Geometry: final body of the model. Coordinates: model frame, mm. Face numbers are marked on the shaded views. Coordinates: 2 decimals unless noted, no trailing zeros. Answer in a Markdown table with one row per item.
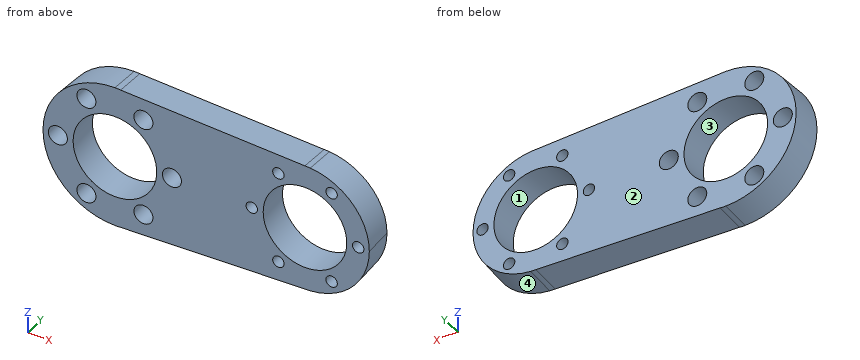
from build123d import *

# Parameters (mm, degrees)
F1_DEPTH = 8
F1_TAPER = -3
F3_D     = 22
F4_D     = 22
F6_D     = 5
F7_D     = 3


# Not quite as in the source:
# - a feature of the source that left no trace in its solid (it failed there, or was rolled back) is left out


with BuildPart() as f1:
    # F0 (on Front) → F1 (new body)
    with BuildSketch(Plane.XZ):
        with BuildLine():
            Line((1.4786393064, 18.4408141307), (0, 18.5))
            ThreePointArc((0, 18.5), (-18.5, 0), (0, -18.5))
            Line((0, -18.5), (1.4786393064, -18.4408141307))
            ThreePointArc((1.4786393064, -18.4408141307), (13.5942051472, -12.5478120171), (18.5, 0))
            ThreePointArc((18.5, 0), (13.5942051472, 12.5478120171), (1.4786393064, 18.4408141307))
        make_face()
        with BuildLine():
            ThreePointArc((1.4786393064, 18.4408141307), (0.7399116781, 18.4851976108), (0, 18.5))
            Line((0, 18.5), (1.4786393064, 18.4408141307))
        make_face()
        with BuildLine():
            Line((1.4786393064, -18.4408141307), (0, -18.5))
            ThreePointArc((0, -18.5), (0.7399116781, -18.4851976108), (1.4786393064, -18.4408141307))
        make_face()
        with BuildLine():
            Line((49.9667920397, 16.4999665827), (1.4786393064, 18.4408141307))
            ThreePointArc((1.4786393064, 18.4408141307), (13.5942051472, 12.5478120171), (18.5, 0))
            Line((18.5, 0), (33.5, 0))
            ThreePointArc((33.5, 0), (38.3210032249, 11.6555151893), (49.9667920397, 16.4999665827))
        make_face()
        with BuildLine():
            ThreePointArc((18.5, 0), (13.5942051472, -12.5478120171), (1.4786393064, -18.4408141307))
            Line((1.4786393064, -18.4408141307), (49.9667920397, -16.4999665827))
            ThreePointArc((49.9667920397, -16.4999665827), (38.3210032249, -11.6555151893), (33.5, 0))
            Line((33.5, 0), (18.5, 0))
        make_face()
        with BuildLine():
            Line((51.3518854576, 16.4445250983), (49.9667920397, 16.4999665827))
            ThreePointArc((49.9667920397, 16.4999665827), (38.3210032249, 11.6555151893), (33.5, 0))
            ThreePointArc((33.5, 0), (38.3210032249, -11.6555151893), (49.9667920397, -16.4999665827))
            Line((49.9667920397, -16.4999665827), (51.3518854576, -16.4445250983))
            ThreePointArc((51.3518854576, -16.4445250983), (62.1358170316, -11.1790851582), (66.5, 0))
            ThreePointArc((66.5, 0), (62.1358170316, 11.1790851582), (51.3518854576, 16.4445250983))
        make_face()
        with BuildLine():
            ThreePointArc((51.3518854576, 16.4445250983), (50.6599212264, 16.4867978691), (49.9667920397, 16.4999665827))
            Line((49.9667920397, 16.4999665827), (51.3518854576, 16.4445250983))
        make_face()
        with BuildLine():
            Line((51.3518854576, -16.4445250983), (49.9667920397, -16.4999665827))
            ThreePointArc((49.9667920397, -16.4999665827), (50.6599212264, -16.4867978691), (51.3518854576, -16.4445250983))
        make_face()
    extrude(amount=F1_DEPTH, taper=F1_TAPER)

    # F3 (through all)
    with Locations(Plane(origin=(0, 0, 0), x_dir=(1, 0, 0), z_dir=(0, 1, 0))):
        with Locations((50, 0)):
            Hole(F3_D / 2)

    # F4 (through all)
    with Locations(Plane(origin=(0, 0, 0), x_dir=(1, 0, 0), z_dir=(0, 1, 0))):
        with Locations((0, 0)):
            Hole(F4_D / 2)

    # F6 (through all)
    with Locations(Plane.XZ.offset(8)):
        with Locations((15, 0), (7.5, 12.9903810568), (-7.5, 12.9903810568), (-15, 0), (-7.5, -12.9903810568), (7.5, -12.9903810568)):
            Hole(F6_D / 2)

    # F7 (through all)
    with Locations(Plane.XZ.offset(8)):
        with Locations((36, 0), (43, 12.124355653), (57, 12.124355653), (64, 0), (57, -12.124355653), (43, -12.124355653)):
            Hole(F7_D / 2)


solid = f1.part
(1) Ray query, probe 1 along Z at (x, y) = (-15, -1.75); probe 2 along Z at (x, y) = (-7.5, -3.75); probe 3 along X at (y, z) = (-5.5, 3). Return the intervals inside material, ascending.
Verdict:
| item | result |
|---|---|
| probe 1 | z = -10.98 to -2.5, 2.5 to 10.98 |
| probe 2 | z = -17.13 to -15.49, -10.49 to -8.05, 8.05 to 10.49, 15.49 to 17.13 |
| probe 3 | x = -18.55 to -10.58, 10.58 to 39.42, 60.58 to 66.52 |
(2) Cut plane A-A on x = 57. State how many separate pieces and enclosed holes the cut face has, then the cut area to 3 significant figures.
Verdict:
| item | result |
|---|---|
| separate pieces | 4 |
| enclosed holes | 0 |
| area | 59.0 mm² |
(3) Pull-direction query (Z, two-part tool) for the marked faces 1, 2, 3 and 4; classes: pulls with the +Z half, pulls with the -Z half, needs draft (parallel to the pull), parting line crosses it, or undercut.
Verdict:
| item | result |
|---|---|
| face 1 | undercut |
| face 2 | needs draft |
| face 3 | undercut |
| face 4 | pulls with the -Z half |
(4) First-contact query: pin 1 Ø1.5 at (x, y) = (22.5, -2.5) entering from +Z; pin 2 Ø3 at (y, z) = (-3, -9.5) entering from -X; pin 3 Ø4.5 at (x, z) = (7.5, -12.99) entering from -Y; pin 4 Ø2 at (x, y) = (34, -2) entering from -Z. Flat tips, straight axial feed; report the tip coordinate or a pass-through.
Verdict:
| item | result |
|---|---|
| pin 1 | stops at z = 17.78 |
| pin 2 | stops at x = -16.86 |
| pin 3 | passes through |
| pin 4 | stops at z = -17.31 |
